Part model, mm, in its own coordinate system. A direction names the side the tool comes from. Round coordinates to 2 decimals unless told otherwise and drop trailing zeros. Loops run counter-clockwise (first coordinate to the right, second up) from the corner with the lowest first, then second, coordinate; pieces in that order, holes last.
(1) Tool access for faces 1 (the face through (3, -3, 10)), 2 (the face through (0, 0, -8)), 3 (the face through (0, 0, 0)): list every direction of +Z, -Z, +X, -X, +Y, -Y with a clear straight run to the whole face (end or side of a thin tool).
(2) Probe probe 1 along Y at (x, z) = (0, -8.4); probe 2 along Y at (x, z) = (0, 3.5); probe 3 along Z at (x, y) = (3.5, -0.5). List the from-to ranges inside material, lowest first.
(3) Mould opens along X. For faces 4 (the face through (-2.1, 0.66, -9.01)), 5 (the face through (-2, 2, -10)), 6 (the face through (6.466, -2.681, 0.14)) say: +X half, -X half, draft (parallel to the pull), parting line (faces both ways), or undercut.
(4) Cut at D-D on x = -2.75. List the corners of the cut face in (y, z), then the cut area to 3 significant figures.
(5) Cut at C-C on z = 2.75. List the corners of the cut face in (x, y), then the cut area to 3 significant figures.
(6) Flat gauge pins, fed straight in: pin 1 (8 mm diameter, centred on y = -5, z = -6, fed in from -X); pin 2 (1 mm diameter, centred on y = -4.5, z = -6, fed in from +X); pin 3 (2.5 mm diameter, centred on x = 0, y = 0, fed in from -Z). Where does each tip first touch, or does it go through?
(7) Cut at A-A on y = 0. List the corners of the cut face in (x, z), then the cut area to 3 significant figures.
Autodesk Inventor part; units mm, degrees
ref_plane "YZ Plane" through (0, 0, 0) normal (1, 0, 0) x (0, 1, 0)
ref_plane "XZ Plane" through (0, 0, 0) normal (0, 1, 0) x (-1, 0, 0)
ref_plane "XY Plane" through (0, 0, 0) normal (0, 0, 1) x (1, 0, 0)
sketch "Sketch1" plane through (0, 0, 0) normal (0, 0, 1) x (1, 0, 0)
  circle A0 centre (0, 0) radius 3.6
  circle A1 centre (0, 0) radius 7
  dimension "d0" = 7.2
  dimension "d1" = 14
extrude "Extrusion1" add sketch "Sketch1" along normal mid plane 20
extrude "Extrusion2" add sketch "Sketch1" against normal blind 10 contours A0
sketch "Sketch2" plane through (0, 0, -10) normal (0, 0, -1) x (-1, 0, 0)
  circle A0 centre (0, 0) radius 2.2
  dimension "d6" = 4.4
extrude "Extrusion3" cut sketch "Sketch2" against normal blind 2
properties part number "Magnet Coupler"
Final values:
1. face 1: +Z, +X, -X, +Y, -Y
1. face 2: -Z
1. face 3: +Z
2. probe 1: y = -7 to -2.2, 2.2 to 7
2. probe 2: y = -7 to -3.6, 3.6 to 7
2. probe 3: z = -10 to 0
3. face 4: undercut
3. face 5: draft
3. face 6: parting line
4. outline: (-6.44, -10) - (6.44, -10) - (6.44, 10) - (2.32, 10) - (2.32, 0) - (-2.32, 0) - (-2.32, 10) - (-6.44, 10) - close
4. area: 211 mm2
5. outline: circle Ø14 at (0, 0); hole circle Ø7.2 at (0, 0)
5. area: 113 mm2
6. pin 1: stops at x = -6.93
6. pin 2: stops at x = 5.74
6. pin 3: stops at z = -8
7. outline: (-7, -10) - (-2.2, -10) - (-2.2, -8) - (2.2, -8) - (2.2, -10) - (7, -10) - (7, 10) - (3.6, 10) - (3.6, 0) - (-3.6, 0) - (-3.6, 10) - (-7, 10) - close
7. area: 199 mm2
